from build123d import *

# Parameters (mm, degrees)
SKETCH_3_R                  = 2
EXTRUDE_4_DEPTH             = 15
EXTRUDE_5_DEPTH             = 7
HOLE_WIZARD_13_0_13_2_D     = 13
HOLE_WIZARD_13_0_13_2_DEPTH = 15
HOLE_WIZARD_13_0_13_2_TIP   = 3.905594024
HOLE_WIZARD_2_D             = 6.6
HOLE_WIZARD_2_DEPTH         = 15
HOLE_WIZARD_2_CBORE_D       = 11
HOLE_WIZARD_2_CBORE_DEPTH   = 6.8
HOLE_WIZARD_2_TIP           = 1.982840043
FILLET_1_R                  = 1


with BuildPart() as part:
    # 草图3 → 凸台-拉伸4 (new body)
    with BuildSketch(Plane.XY):
        with BuildLine():
            ThreePointArc((-28.916190476, 24.475919449), (-31.903967114, 21.541687531), (-33, 17.5))
            Line((-33, 17.5), (-33, -17.5))
            ThreePointArc((-33, -17.5), (-31.903967114, -21.541687531), (-28.916190476, -24.475919449))
            ThreePointArc((-28.916190476, -24.475919449), (-28.191496301, -25.08958226), (-27.747936508, -25.929236))
            ThreePointArc((-27.747936508, -25.929236), (-20.506096654, -38.006096654), (-8.429236, -45.247936508))
            ThreePointArc((-8.429236, -45.247936508), (-7.58958226, -45.691496301), (-6.975919449, -46.416190476))
            ThreePointArc((-6.975919449, -46.416190476), (0, -50.5), (6.975919449, -46.416190476))
            ThreePointArc((6.975919449, -46.416190476), (7.58958226, -45.691496301), (8.429236, -45.247936508))
            ThreePointArc((8.429236, -45.247936508), (20.506096654, -38.006096654), (27.747936508, -25.929236))
            ThreePointArc((27.747936508, -25.929236), (28.191496301, -25.08958226), (28.916190476, -24.475919449))
            ThreePointArc((28.916190476, -24.475919449), (31.903967114, -21.541687531), (33, -17.5))
            Line((33, -17.5), (33, 17.5))
            ThreePointArc((33, 17.5), (31.903967114, 21.541687531), (28.916190476, 24.475919449))
            ThreePointArc((28.916190476, 24.475919449), (28.191496301, 25.08958226), (27.747936508, 25.929236))
            ThreePointArc((27.747936508, 25.929236), (20.506096654, 38.006096654), (8.429236, 45.247936508))
            ThreePointArc((8.429236, 45.247936508), (7.58958226, 45.691496301), (6.975919449, 46.416190476))
            ThreePointArc((6.975919449, 46.416190476), (0, 50.5), (-6.975919449, 46.416190476))
            ThreePointArc((-6.975919449, 46.416190476), (-7.58958226, 45.691496301), (-8.429236, 45.247936508))
            ThreePointArc((-8.429236, 45.247936508), (-20.506096654, 38.006096654), (-27.747936508, 25.929236))
            ThreePointArc((-27.747936508, 25.929236), (-28.191496301, 25.08958226), (-28.916190476, 24.475919449))
        make_face()
        with Locations((-17.67766953, -35.17766953)):
            Circle(SKETCH_3_R, mode=Mode.SUBTRACT)
        with Locations((17.67766953, 35.17766953)):
            Circle(SKETCH_3_R, mode=Mode.SUBTRACT)
    extrude(amount=EXTRUDE_4_DEPTH)

    # 草图3<6> → 凸台-拉伸5 (add)
    with BuildSketch(Plane.XY):
        with BuildLine():
            Line((14, -17.5), (14, 17.5))
            ThreePointArc((14, 17.5), (0, 31.5), (-14, 17.5))
            Line((-14, 17.5), (-14, -17.5))
            ThreePointArc((-14, -17.5), (0, -31.5), (14, -17.5))
        make_face()
    extrude(amount=-EXTRUDE_5_DEPTH)

    # Ø13.0 (13) 直径孔2
    with Locations(Plane(origin=(0, 17.5, 15), x_dir=(1, 0, 0), z_dir=(0, 0, 1))):
        with Locations((0, 0), (0, -35)):
            Hole(HOLE_WIZARD_13_0_13_2_D / 2, depth=HOLE_WIZARD_13_0_13_2_DEPTH)
            with Locations((0, 0, -(HOLE_WIZARD_13_0_13_2_DEPTH + HOLE_WIZARD_13_0_13_2_TIP / 2))):  # 118° drill point
                Cone(0, HOLE_WIZARD_13_0_13_2_D / 2, HOLE_WIZARD_13_0_13_2_TIP, mode=Mode.SUBTRACT)

    # 打孔尺寸(%根据)开槽圆柱头螺钉的类型2
    with Locations(Plane(origin=(0, 0, 0), x_dir=(-1, 0, 0), z_dir=(0, 0, -1))):
        with Locations((0, 42.5), (-25, 17.5), (25, 17.5), (-25, -17.5), (25, -17.5), (0, -42.5)):
            CounterBoreHole(HOLE_WIZARD_2_D / 2, HOLE_WIZARD_2_CBORE_D / 2, HOLE_WIZARD_2_CBORE_DEPTH, depth=HOLE_WIZARD_2_DEPTH)
            with Locations((0, 0, -(HOLE_WIZARD_2_DEPTH + HOLE_WIZARD_2_TIP / 2))):  # 118° drill point
                Cone(0, HOLE_WIZARD_2_D / 2, HOLE_WIZARD_2_TIP, mode=Mode.SUBTRACT)

    # 圆角1
    fillet_1_edges = [part.edges().sort_by_distance(p)[0] for p in [
        (14, 0, -7),
        (0, -31.5, -7),
        (-14, 0, 0),
        (0, 31.5, -7),
        (-14, 0, -7),
        (14, 0, 0),
        (0, 31.5, 0),
        (0, -31.5, 0),
    ]]
    fillet(fillet_1_edges, radius=FILLET_1_R)


solid = part.part
Can you work these out from the model? Positions are in its coordinate system, mm. A direction names the side the tool comes from. Give positions to 0.01 mm unless a question says otherwise; leave off trailing zeros. Order: outer loops, then holes, each group sorted by start corner. A loop starts at its lowest first (then second) coordinate and runs counter-clockwise, first axis right, second up. Notation, with made-up numbers: M -35.75,-4 L 20.25,-4 A22 cw 20.25,15 Z; hole C 33,59.25 d5. An arc over 180 degrees is marked long. Use one line per item in the form item = value. Start each with the question number.
Item 1: If we section it at D-D (y = -6.5): Write out the boundary of the cut face in (x, z).
Item 2: If we section it at A-A (x = 25): Write out the boundary of the cut face in (y, z), then the cut area to 3 significant figures.
Item 3: If I drill on line 1 along Y through (x, z) = (0, 7.5); line 2 along X through (y, z) = (-17.5, 12); line 3 along Y through (x, z) = (-25, 10.5), over which ranges is the centre line in solid material (lowest first)?
Item 4: If we section it at B-B (z = 1): State how many separate pieces and enclosed holes the cut face has, then the cut area to 3 significant figures.
Item 5: Will these pins go through, and if not, where does the flat tip stop? pin 1 Ø4 at (x, z) = (26, 9) entering from -Y; pin 2 Ø2 at (y, z) = (-30, -1.5) entering from +X; pin 3 Ø6 at (x, z) = (-8.5, 2.5) entering from -Y.
Item 6: We'd pull the mould along Y, two halves only. Please class faces 1 (the cylindrical face through (-21.95, 16.24, 10.96)), 2 (the cylindrical face through (31.934, 21.49, 7.395)), 3 (the flat face through (-22, 1, 0)): +Y half, -Y half, draft (parallel to the pull), parting line (faces both ways), or undercut.
Item 7: For faces 4 (the cylindrical face through (0.846, -11.055, 7.395)), 5 (the cylindrical face through (0.1, 50.5, 7.4)), 6 (the cylindrical face through (-30.08, -19.61, 3.35)), which set-ups out of +Z, -Z, +X, -X, +Y, -Y let a thin tool reach every point of the face, with its end or its side?
Item 8: If we section it at C-C (y = -41.5): Write out the boundary of the cut face in (x, z), then the cut area to 3 significant figures.
Outcome:
q1.outline = M -33,0 L -15,0 A1 cw -14,-1 L -14,-6 A1 ccw -13,-7 L 13,-7 A1 ccw 14,-6 L 14,-1 A1 cw 15,0 L 33,0 L 33,15 L -33,15 Z
q2.outline = M -32.2,0 L -23,0 L -23,6.8 L -20.8,6.8 L -20.8,15 L -32.2,15 Z; M -14.2,6.8 L -12,6.8 L -12,0 L 12,0 L 12,6.8 L 14.2,6.8 L 14.2,15 L -14.2,15 Z; M 20.8,6.8 L 23,6.8 L 23,0 L 32.2,0 L 32.2,15 L 20.8,15 Z
q2.area = 708 mm2
q3.line_1 = -50.5 to -45.8, -39.2 to -24, -11 to 11, 24 to 39.2, 45.8 to 50.5
q3.line_2 = -33 to -28.3, -21.7 to -6.5, 6.5 to 21.7, 28.3 to 33
q3.line_3 = -32.2 to -20.8, -14.2 to 14.2, 20.8 to 32.2
q4.separate_pieces = 1
q4.enclosed_holes = 10
q4.area = 4,270 mm2
q5.pin_1 = -33.78
q5.pin_2 = 7.98
q5.pin_3 = -48.31
q6.face_1 = undercut
q6.face_2 = +Y half
q6.face_3 = draft
q7.face_4 = +Z
q7.face_5 = +Z, -Z, +Y
q7.face_6 = -Z
q8.outline = M -16.28,0 L -5.41,0 L -5.41,6.8 L -3.14,6.8 L -3.14,15 L -16.28,15 Z; M 3.14,6.8 L 5.41,6.8 L 5.41,0 L 16.28,0 L 16.28,15 L 3.14,15 Z
q8.area = 363 mm2
